```python
from build123d import *

# Parameters (mm, degrees)
SKETCH1_W           = 30
SKETCH1_H           = 22
BOSS_EXTRUDE1_DEPTH = 66
SKETCH2_R           = 8
BOSS_EXTRUDE2_DEPTH = 20.2
BOSS_EXTRUDE3_START = 20.2
SKETCH3_R           = 8
BOSS_EXTRUDE3_DEPTH = 20.2
SHELL1_T            = -2


with BuildPart() as part:
    # Sketch1 → Boss-Extrude1 (new body)
    with BuildSketch(Plane(origin=(0, 0, 0), x_dir=(1, 0, 0), z_dir=(0, 1, 0))):
        Rectangle(SKETCH1_W, SKETCH1_H)
    extrude(amount=BOSS_EXTRUDE1_DEPTH)

    # Sketch2 → Boss-Extrude2 (add)
    with BuildSketch(Plane.ZY.offset(15)):
        with Locations(Location((0, 9, 0), (0, 0, 180))):
            Circle(SKETCH2_R)
    extrude(amount=BOSS_EXTRUDE2_DEPTH)

    # Sketch3 → Boss-Extrude3 (add)
    with BuildSketch(Plane(origin=(15, 0, 0), x_dir=(0, 0, -1), z_dir=(1, 0, 0)).offset(BOSS_EXTRUDE3_START)):
        with Locations((0, 9)):
            Circle(SKETCH3_R)
    extrude(amount=-BOSS_EXTRUDE3_DEPTH)

    # Shell1
    shell1_openings = [part.faces().sort_by_distance(p)[0] for p in [
        (-35.2, 9, 0),
        (35.2, 9, 0),
    ]]
    offset(amount=SHELL1_T, openings=shell1_openings, kind=Kind.INTERSECTION)


solid = part.part
```
Part model, mm, in its own coordinate system. A direction names the side the tool comes from. Round coordinates to 2 decimals unless told otherwise and drop trailing zeros. Loops run counter-clockwise (first coordinate to the right, second up) from the corner with the lowest first, then second, coordinate; pieces in that order, holes last.
Item 1: Cut at C-C, the plane y = 9. Give the cut face in (x, z).
Item 2: Drop flat-ended pins along their axis: P1, Ø3, axis at x = -25, z = -1.5, coming from the -Y side; P2, Ø1.5, axis at y = 22, z = -4, coming from the +X side; P3, Ø12, axis at y = 53, z = 2, coming from the -X side. Give the stop position or say it passes through.
Item 3: Cut at A-A, the plane z = 0. Give the cut face in (x, y), then the cut area to 3 significant figures.
Item 4: Drill centre lines: line 1 (X direction, y = 26.5, z = -3.75); line 2 (Y direction, x = -24.25, z = 0); line 3 (Z direction, x = -1, y = 37). Where is each one in solid material? Low to high.
Item 5: Cut at D-D, the plane y = 32.5. Give the cut face in (x, z), then the cut area to 3 significant figures.
Item 6: 3-axis set-ups, long thin cutter, end or side, ignore diameter. For faces 1 (the face through (-24.96, 16.81, 1.73)), 2 (the face through (25.24, 1.19, 1.73)), 3 (the face through (0, 2, 0)), 4 (the face through (-23.94, 3.05, 0.78)): which of +Z, -Z, +X, -X, +Y, -Y reach the whole face in a straight line?
Item 7: Mould opens along Z. For faces 5 (the face through (0, 0, 0)), 6 (the face through (0, 33, -11)), 7 (the face through (0, 33, 9)), 8 (the face through (24.255, 3.143, 1.301)) say: +Z half, -Z half, draft (parallel to the pull), parting line (faces both ways), or undercut.
Item 8: Cut at B-B, the plane x = 10.5. Give the cut face in (y, z).
A:
1. outline: (-35.2, -8) - (-15, -8) - (-15, -11) - (15, -11) - (15, -8) - (35.2, -8) - (35.2, -6) - (13, -6) - (13, -9) - (-13, -9) - (-13, -6) - (-35.2, -6) - close; (-35.2, 6) - (-13, 6) - (-13, 9) - (13, 9) - (13, 6) - (35.2, 6) - (35.2, 8) - (15, 8) - (15, 11) - (-15, 11) - (-15, 8) - (-35.2, 8) - close
2. P1: stops at y = 1
2. P2: stops at x = 15
2. P3: stops at x = -15
3. outline: (-35.2, 1) - (-15, 1) - (-15, 0) - (15, 0) - (15, 1) - (35.2, 1) - (35.2, 3) - (13, 3) - (13, 2) - (-13, 2) - (-13, 3) - (-35.2, 3) - close; (-35.2, 15) - (-13, 15) - (-13, 64) - (13, 64) - (13, 15) - (35.2, 15) - (35.2, 17) - (15, 17) - (15, 66) - (-15, 66) - (-15, 17) - (-35.2, 17) - close
3. area: 482 mm2
4. line 1: x = -15 to -13, 13 to 15
4. line 2: y = 1 to 3, 15 to 17
4. line 3: z = -11 to -9, 9 to 11
5. outline: (-15, -11) - (15, -11) - (15, 11) - (-15, 11) - close; hole (-13, -9) - (13, -9) - (13, 9) - (-13, 9) - close
5. area: 192 mm2
6. face 1: -X
6. face 2: +X
6. face 3: none
6. face 4: +X, -X
7. face 5: draft
7. face 6: -Z half
7. face 7: undercut
7. face 8: undercut
8. outline: (0, -11) - (66, -11) - (66, 11) - (0, 11) - close; hole (2, -9) - (64, -9) - (64, 9) - (2, 9) - close
